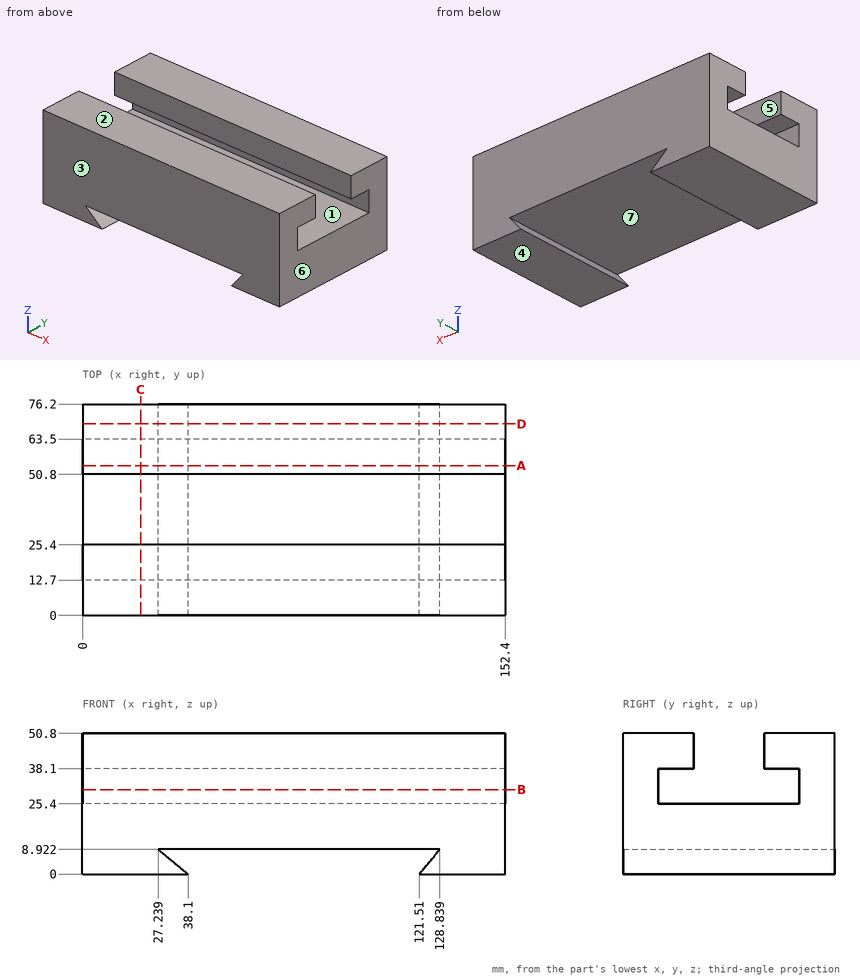
Source: three-view drawing plus pictorial views. Frame: mm from the lowest corner of the part. A direction names the side the tool comes from. Give positions to 0.01 mm unless a question says otherwise; leave off trailing zeros. Write each loop counter-clockwise with the first axis right and the second up, starting at its lowest first coordinate (ties: lowest second). Pieces come first, ordered by that corner, then holes. Notation, with made-up numbers: (74.25, 4.5) - (106.25, 4.5) arc R28 cw to (106.25, 29.5) - close; hole circle Ø3 at (46.25, 6.5). An arc over 180 degrees is marked (long way). Write item = value, one per line. Start each with the question number.
Q1. Cut plane B-B, the plane z = 30.5. Return loops of the section in (x, y).
Q2. Cut plane D-D, the plane y = 69. Return loops of the section in (x, z).
Q3. Material intervals for probe 1 along Z at (x, y) = (38.5, 24); probe 2 along Y at (x, z) = (79.5, 44); probe 3 along Y at (x, z) = (118, 35), sorted ascending.
Q4. Cut plane A-A, the plane y = 54. Return loops of the section in (x, z).
Q5. Reachability of the marked faces 5, 6 and 7 from +Z, -Z, +X, -X, +Y, -Y: full face, straight path, thin tool, end or side. Return the list, or none.
Q6. Cut plane C-C, the plane x = 21. Return loops of the section in (y, z).
Q7. Draft query along Z for the marked faces 1, 2, 3 and 4. Return one class per face: +Z half, -Z half, draft (parallel to the pull), parting line (faces both ways), or undercut.
Q8. Pin query (flat end, axial travel): pin 1 Ø3 at (x, z) = (111.5, 32.5) entering from -Y; pin 2 Ø10 at (x, y) = (80.5, 17.5) entering from -Z; pin 3 Ø1.5 at (x, y) = (66.5, 50) entering from +Z. Return the tip coordinate at first contact, or that it passes through.
Computed values:
q1.outline = (0, 0) - (152.4, 0) - (152.4, 12.7) - (0, 12.7) - close; (0, 63.5) - (152.4, 63.5) - (152.4, 76.2) - (0, 76.2) - close
q2.outline = (0, 0) - (38.1, 0) - (27.24, 8.92) - (128.84, 8.92) - (121.51, 0) - (152.4, 0) - (152.4, 50.8) - (0, 50.8) - close
q3.probe_1 = 8.92 to 25.4, 38.1 to 50.8
q3.probe_2 = 0 to 25.4, 50.8 to 76.2
q3.probe_3 = 0 to 12.7, 63.5 to 76.2
q4.outline = (0, 0) - (38.1, 0) - (27.24, 8.92) - (128.84, 8.92) - (121.51, 0) - (152.4, 0) - (152.4, 25.4) - (0, 25.4) - close; (0, 38.1) - (152.4, 38.1) - (152.4, 50.8) - (0, 50.8) - close
q5.face_5 = +Z, +X, -X
q5.face_6 = +Z, -Z, +X, +Y, -Y
q5.face_7 = +Y, -Y
q6.outline = (0, 0) - (76.2, 0) - (76.2, 50.8) - (50.8, 50.8) - (50.8, 38.1) - (63.5, 38.1) - (63.5, 25.4) - (12.7, 25.4) - (12.7, 38.1) - (25.4, 38.1) - (25.4, 50.8) - (0, 50.8) - close
q7.face_1 = undercut
q7.face_2 = +Z half
q7.face_3 = draft
q7.face_4 = -Z half
q8.pin_1 = 0
q8.pin_2 = 8.92
q8.pin_3 = 25.4
